Job drawing, mm, ordinate dimensions from the low corner. One solid piece. A direction names the side the tool comes from. Give positions to 0.01 mm unless a question says otherwise; leave off trailing zeros. Order: outer loops, then holes, each group sorted by start corner. A loop starts at its lowest first (then second) coordinate and runs counter-clockwise, first axis right, second up. Notation, with made-up numbers: M 87,-23 L 129,-23 A15 ccw 129,1 Z; hole C 24,-9 d2. An arc over 180 degrees is marked long. One line per question, with ' | ' between items.
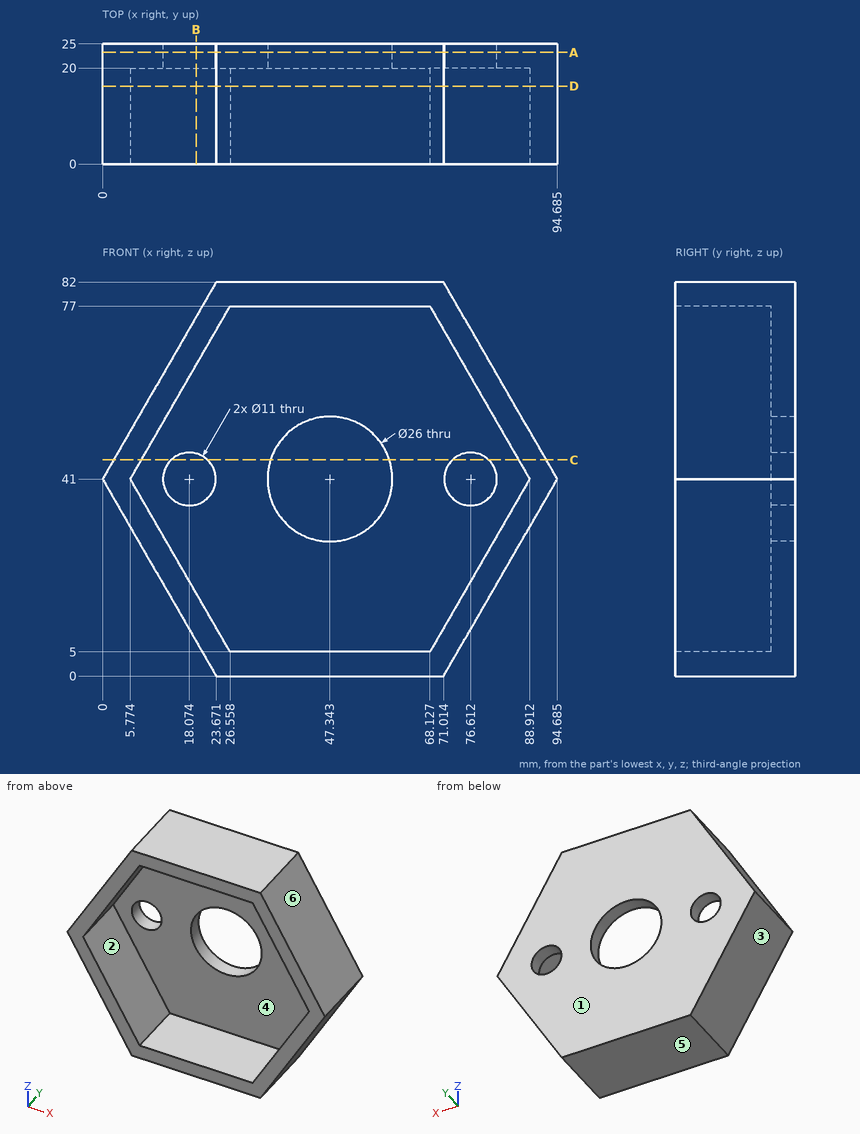
1. Slice it at C-C on z = 45. Give the cut face in (x, y).
Worked out:
outline: M 2.31,0 L 8.08,0 L 8.08,20 L 14.3,20 L 14.3,25 L 2.31,25 Z; M 21.85,20 L 34.97,20 L 34.97,25 L 21.85,25 Z; M 59.71,20 L 72.84,20 L 72.84,25 L 59.71,25 Z; M 80.39,20 L 86.6,20 L 86.6,0 L 92.38,0 L 92.38,25 L 80.39,25 Z
2. Mould opens along X. For the marked faces 3, 4, 5 and 6 say: released by +X, released by -X, zero draft, split by the parting line, or undercut.
Worked out:
face 3: released by -X | face 4: undercut | face 5: zero draft | face 6: released by +X
3. Drop flat-ended pins along their axis: pin 1 (21.5 mm diameter, centred on x = 30.5, z = 46.5, fed in from -Y); pin 2 (5 mm diameter, centred on x = 74, y = 4.5, fed in from -Z); pin 3 (8 mm diameter, centred on x = 83.5, y = 9, fed in from +Z) (1 decimal). Give the stop position or say it passes through.
Worked out:
pin 1: stops at y = 20 | pin 2: stops at z = 0.84 | pin 3: stops at z = 67.3
4. Slice it at B-B on x = 19.5. Give the cut face in (y, z) (1 decimal).
Worked out:
outline: M 0,7.2 L 25,7.2 L 25,35.7 L 20,35.7 L 20,17.2 L 0,17.2 Z; M 0,64.8 L 20,64.8 L 20,46.3 L 25,46.3 L 25,74.8 L 0,74.8 Z
5. Tool access for the marked faces 1 and 2: list every direction of +Z, -Z, +X, -X, +Y, -Y with a clear straight run to the whole face (end or side of a thin tool).
Worked out:
face 1: +Z, -Z, +X, -X, +Y | face 2: -Y
6. Probe L1, parallel to Z at x = 62.5, y = 1.5; L2, parallel to Y at x = 68, z = 8.5; L3, parallel to Z at x = 22, y = 3 (1 decimal). List the from-to ranges inside material, lowest first. Write a range as from..to.
Worked out:
L1: z = 0..5, 77..82 | L2: y = 20..25 | L3: z = 2.9..12.9, 69.1..79.1
7. Slice it at D-D on y = 16.25. Give the cut face in (x, z) (1 decimal).
Worked out:
outline: M 0,41 L 23.7,0 L 71,0 L 94.7,41 L 71,82 L 23.7,82 Z; hole M 5.8,41 L 26.6,5 L 68.1,5 L 88.9,41 L 68.1,77 L 26.6,77 Z
8. Slice it at A-A on y = 23.25. Give the cut face in (x, z) (1 decimal).
Worked out:
outline: M 0,41 L 23.7,0 L 71,0 L 94.7,41 L 71,82 L 23.7,82 Z; hole C 18.1,41 d11; hole C 47.3,41 d26; hole C 76.6,41 d11
